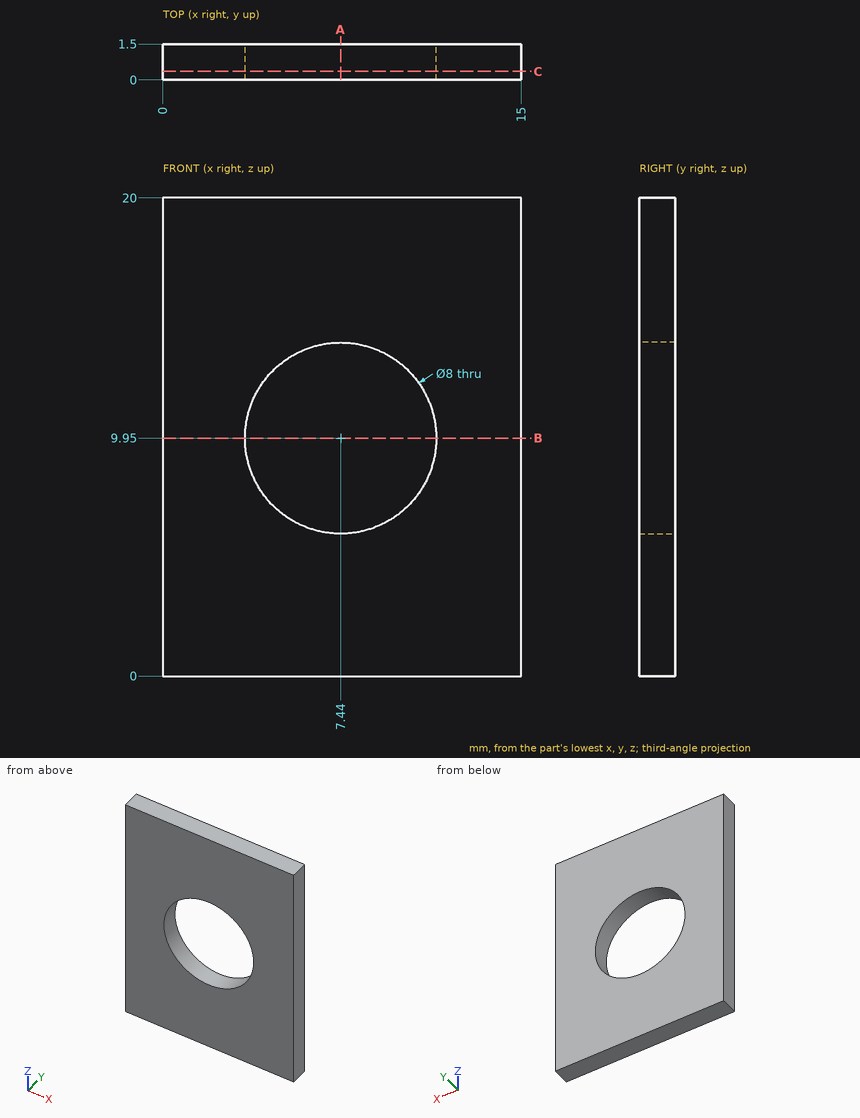
Geometry: see drawing. Coordinates: mm, zero at the bounding-box minimum. Give positions to 0.01 mm unless a question says otherwise; leave off trailing zeros. Order: outer loops, then holes, each group sorted by start corner. A loop starts at its lowest first (then second) coordinate and runs counter-clockwise, first axis right, second up. Notation, with made-up numbers: (50, 72.25) - (71, 72.25) arc R25 ccw to (71, 110.25) - close; hole circle Ø4 at (2, 37). An arc over 180 degrees is marked (long way). One line per item, written item: value.
1. Cut plane B-B, the plane z = 9.95. Output: boundary loops of the cut face in (x, y), and give its area (3 significant figures).
Determined:
outline: (0, 0) - (3.44, 0) - (3.44, 1.5) - (0, 1.5) - close; (11.44, 0) - (15, 0) - (15, 1.5) - (11.44, 1.5) - close
area: 10.5 mm2
2. Cut plane C-C, the plane y = 0.35. Output: boundary loops of the cut face in (x, z).
Determined:
outline: (0, 0) - (15, 0) - (15, 20) - (0, 20) - close; hole circle Ø8 at (7.44, 9.95)
3. Pin query (flat end, axial travel): pin 1 Ø2 at (x, z) = (3.5, 16.5) entering from -Y. Return the tip coordinate at first contact, or that it passes through.
Determined:
pin 1: y = 0
4. Cut plane A-A, the plane x = 7.44. Output: boundary loops of the cut face in (y, z), and give its area (3 significant figures).
Determined:
outline: (0, 0) - (1.5, 0) - (1.5, 5.95) - (0, 5.95) - close; (0, 13.95) - (1.5, 13.95) - (1.5, 20) - (0, 20) - close
area: 18.0 mm2
5. Line query: probe 1 along X at (y, z) = (1.3, 10); probe 2 along Z at (x, y) = (7.25, 1.05); probe 3 along Z at (x, y) = (4.75, 1.1). Output: solid intervals per line, ascending.
Determined:
probe 1: 0 to 3.44, 11.44 to 15
probe 2: 0 to 5.95, 13.95 to 20
probe 3: 0 to 6.99, 12.91 to 20
